```python
from build123d import *

# Parameters (mm, degrees)
SKETCH1_W               = 30
SKETCH1_H               = 30
BOSS_EXTRUDE1_DEPTH     = 15
FILLET1_R               = 4
CHAMFER2_SIZE           = 3
FILLET2_R               = 1
SKETCH3_R               = 10
BOSS_EXTRUDE2_DEPTH     = 2.5
FILLET3_R               = 5
SKETCH5_W               = 5
SKETCH5_H               = 15
BOSS_EXTRUDE3_DEPTH     = 20
CHAMFER3_SIZE           = 2
CUT_EXTRUDE1_DEPTH      = 77.075620293
CUT_EXTRUDE1_DEPTH_BACK = 10
SKETCH6_R               = 5
SKETCH7_R               = 0.75
BOSS_EXTRUDE4_DEPTH     = 40
CIRPATTERN1_COUNT       = 8
SKETCH8_R               = 5
CUT_EXTRUDE2_DEPTH      = 10
CUT_EXTRUDE3_DEPTH      = 1
LPATTERN1_COUNT         = 2
LPATTERN1_PITCH         = 5
LPATTERN1_COL_COUNT     = 2
LPATTERN1_COL_PITCH     = 5


with BuildPart() as part:
    # Sketch1 → Boss-Extrude1 (new, symmetric)
    with BuildSketch(Plane.XY):
        Rectangle(SKETCH1_W, SKETCH1_H)
    extrude(amount=BOSS_EXTRUDE1_DEPTH, both=True)

    # Sketch2 → Revolve1 (revolve)
    with BuildSketch(Plane(origin=(0, 0, 0), x_dir=(0, 0, -1), z_dir=(1, 0, 0))):
        Polygon((-55, 0), (-55, 15), (-52, 15), (-52, 9), (-15, 9), (-15, 0), align=None)
    revolve(axis=Axis((0, 0, 15), (0, 0, 1)))

    # Fillet1
    fillet1_edges = [part.edges().sort_by_distance(p)[0] for p in [
        (15, -15, 0),
        (-15, -15, 0),
        (-15, 15, 0),
        (15, 15, 0),
    ]]
    fillet(fillet1_edges, radius=FILLET1_R)

    # Chamfer2
    # the kernel refuses this chamfer: 3 mm, written as the material it takes off along each edge
    with BuildSketch(Plane(origin=(15, 18.715048964, 15), x_dir=(-0.9996219169112969, 0, 0.02749587661058621), z_dir=(0, -1, 0))) as chamfer2_piece_1:
        Polygon((CHAMFER2_SIZE * 0.999621916911, CHAMFER2_SIZE * 0.0274958766106), (-CHAMFER2_SIZE * 0.0274958766106, CHAMFER2_SIZE * 0.999621916911), (0, 0), align=None)
    extrude(amount=37.430097928, mode=Mode.SUBTRACT)

    # Fillet2
    fillet2_edges = [part.edges().sort_by_distance(p)[0] for p in [
        (13.828427125, 13.828427125, -15),
        (15, 0, -15),
        (13.828427125, -13.828427125, -15),
        (0, -15, -15),
        (-13.828427125, -13.828427125, -15),
        (-15, 0, -15),
        (-13.828427125, 13.828427125, -15),
        (11.50401717, 14.968118785, 15),
        (11.50401717, -14.968118785, 15),
        (0, -15, 15),
        (-13.828427125, -13.828427125, 15),
        (-15, 0, 15),
        (-13.828427125, 13.828427125, 15),
        (0, 15, -15),
        (0, 15, 15),
    ]]
    fillet(fillet2_edges, radius=FILLET2_R)

    # Sketch3 → Boss-Extrude2 (add, symmetric)
    with BuildSketch(Plane(origin=(0, 0, -15), x_dir=(-1, 0, 0), z_dir=(0, 0, -1))):
        with Locations(Location((0, 0, 0), (0, 0, 180))):
            Circle(SKETCH3_R)
    extrude(amount=BOSS_EXTRUDE2_DEPTH, both=True)

    # Fillet3
    # the kernel refuses this fillet: 5 mm, written as the material it takes off along each edge
    with BuildSketch(Plane(origin=(0, 0, -17.5), x_dir=(1, 0, 0), z_dir=(0, 1, 0))) as fillet3_piece_1:
        with BuildLine():
            CenterArc((5.669872981, -5), FILLET3_R, 30, 60)
            Line((5.669872981, 0), (5.669872981, 0.1))
            Line((5.669872981, 0.1), (10, 0.1))
            Line((10, 0.1), (10.1, 0))
            ThreePointArc((10.1, 0), (10.1, -1.25), (10.08660254, -2.45))
            Line((10.08660254, -2.45), (10, -2.5))
        make_face()
    revolve(axis=Axis((0, 0, -17.5), (0, 0, -1)), mode=Mode.SUBTRACT)

    # Sketch5 → Boss-Extrude3 (add)
    with BuildSketch(Plane(origin=(0, 0, -15), x_dir=(-1, 0, 0), z_dir=(0, 0, -1))):
        with Locations((-15, 0)):
            Rectangle(SKETCH5_W, SKETCH5_H)
    extrude(amount=-BOSS_EXTRUDE3_DEPTH)

    # Chamfer3
    chamfer3_edges = [part.edges().sort_by_distance(p)[0] for p in [
        (17.5, 7.5, -5),
        (17.5, 0, 5),
        (17.5, -7.5, -5),
    ]]
    chamfer(chamfer3_edges, length=CHAMFER3_SIZE)

    # Sketch6 → Cut-Extrude1 (cut, two sides: drawn at the far end of the back side and taken through both)
    with BuildSketch(Plane.XY.offset(55).offset(-CUT_EXTRUDE1_DEPTH_BACK)):
        with Locations(Location((0, 0, 0), (0, 0, 180))):
            Circle(SKETCH6_R)
    extrude(amount=CUT_EXTRUDE1_DEPTH + CUT_EXTRUDE1_DEPTH_BACK, mode=Mode.SUBTRACT)

    # Sketch7 → Boss-Extrude4 (add)
    with BuildSketch(Plane.XY.offset(55)):
        with Locations((0, 11)):
            Circle(SKETCH7_R)
    boss_extrude4 = extrude(amount=-BOSS_EXTRUDE4_DEPTH)

    # CirPattern1: Boss-Extrude4 ×8 about axis
    cirpattern1_axis = Axis((0, 0, 0), (0, 0, 1))
    for i in range(1, CIRPATTERN1_COUNT):
        add(boss_extrude4.rotate(cirpattern1_axis, i * 360 / CIRPATTERN1_COUNT))

    # Sketch8 → Cut-Extrude2 (cut)
    with BuildSketch(Plane.ZY.offset(15)):
        with Locations(Location((0, 0, 0), (0, 0, 270))):
            Circle(SKETCH8_R)
    extrude(amount=-CUT_EXTRUDE2_DEPTH, mode=Mode.SUBTRACT)

    # Sketch9 → Cut-Extrude3 (cut)
    with BuildSketch(Plane(origin=(0, 15, 0), x_dir=(1, 0, 0), z_dir=(0, 1, 0))):
        with BuildLine():
            Line((1, 10), (1, -10))
            ThreePointArc((1, -10), (0, -11), (-1, -10))
            Line((-1, -10), (-1, 10))
            ThreePointArc((-1, 10), (0, 11), (1, 10))
        make_face()
    cut_extrude3 = extrude(amount=-CUT_EXTRUDE3_DEPTH, mode=Mode.SUBTRACT)

    # LPattern1: Cut-Extrude3 ×2
    with Locations(*[(i * LPATTERN1_PITCH, 0, 0) for i in range(1, LPATTERN1_COUNT)]):
        add(cut_extrude3, mode=Mode.SUBTRACT)

    # LPattern1 col: Cut-Extrude3 ×2
    with Locations(*[(-i * LPATTERN1_COL_PITCH, 0, 0) for i in range(1, LPATTERN1_COL_COUNT)]):
        add(cut_extrude3, mode=Mode.SUBTRACT)


solid = part.part
```
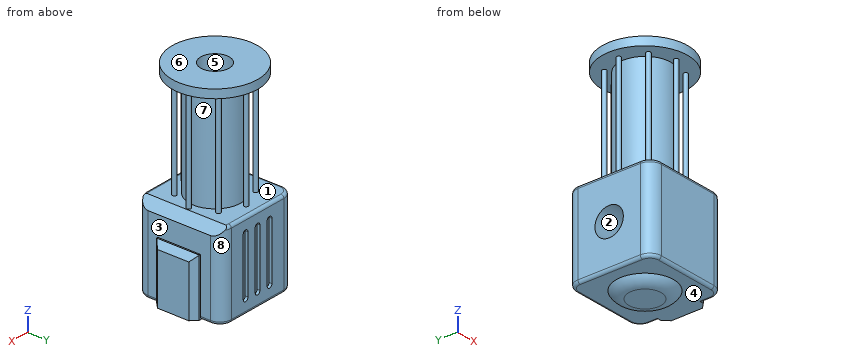
Part model, mm, in its own coordinate system. Face numbers are marked on the shaded views. A direction names the side the tool comes from. Round coordinates to 2 decimals unless told otherwise and drop trailing zeros. Order: outer loops, then holes, each group sorted by start corner. A loop starts at its lowest first (then second) coordinate and runs counter-clockwise, first axis right, second up. Notation, with made-up numbers: M -0.5,38.25 L 3.5,38.25 A29 cw 3.5,66.25 Z; hole C 70,77.5 d9. An arc over 180 degrees is marked long. Put each result on its own line as item: value. Start each with the question number.
1. Tool access for the marked faces 1, 2, 3 and 4: list every direction of +Z, -Z, +X, -X, +Y, -Y with a clear straight run to the whole face (end or side of a thin tool).
2. Drill centre lines: probe 1 along Z at (x, y) = (-12, 0); probe 2 along Z at (x, y) = (7, 8); probe 3 along Y at (x, z) = (0, 49.75). Where is each one in solid material? Low to high. Write a range as [from, to].
3. Two-plate mould, pull along X, no slides. Class the marked faces 5, 6, 7 and 8: +X half, -X half, draft (parallel to the pull), parting line (faces both ways), or undercut.
4. Slice it at A-A on z = -8. List the corners of the cut face in (x, y).
5. Drop flat-ended pins along their axis: pin 1 (1 mm diameter, centred on x = 5, z = -5, fed in from +Y); pin 2 (12 mm diameter, centred on y = 2, z = 23, fed in from -X); pin 3 (1.1 mm diameter, centred on y = 14.5, z = -2, fed in from -X). Give the stop position or say it passes through.
Findings:
1. face 1: none
1. face 2: -X
1. face 3: +Z, +X
1. face 4: -Z
2. probe 1: [-15, -5], [5, 15], [52, 55]
2. probe 2: [-15, 15], [52, 55]
2. probe 3: [-11.75, -10.25], [-9, -5], [5, 9], [10.25, 11.75]
3. face 5: undercut
3. face 6: draft
3. face 7: undercut
3. face 8: +X half
4. outline: M -15,-11 A4 ccw -11,-15 L 11,-15 A4 ccw 15,-11 L 15,-7.5 L 15.5,-7.5 L 17.5,-5.5 L 17.5,5.5 L 15.5,7.5 L 15,7.5 L 15,11 A4 ccw 11,15 L 6,15 L 6,14 L 4,14 L 4,15 L 1,15 L 1,14 L -1,14 L -1,15 L -4,15 L -4,14 L -6,14 L -6,15 L -11,15 A4 ccw -15,11 Z
5. pin 1: y = 14
5. pin 2: x = -11.75
5. pin 3: x = -13.7
